```python
from build123d import *

# Parameters (mm, degrees)
SKETCH1_R           = 7.62
BOSS_EXTRUDE1_DEPTH = 2.54
SKETCH2_R           = 6.35
BOSS_EXTRUDE2_DEPTH = 2.54
SKETCH4_R           = 3.175
CUT_EXTRUDE1_DEPTH  = 8.62


with BuildPart() as part:
    # Sketch1 → Boss-Extrude1 (new body)
    with BuildSketch(Plane.XY):
        Circle(SKETCH1_R)
    boss_extrude1 = extrude(amount=BOSS_EXTRUDE1_DEPTH)

    # Sketch2 → Boss-Extrude2 (add)
    with BuildSketch(Plane.XY.offset(2.54)):
        Circle(SKETCH2_R)
    extrude(amount=BOSS_EXTRUDE2_DEPTH)

    # Mirror1: Boss-Extrude1 across plane
    add(boss_extrude1.mirror(Plane.XY.offset(3.81)))

    # Sketch4 → Cut-Extrude1 (cut, through all)
    with BuildSketch(Plane.XY.offset(7.62)):
        Circle(SKETCH4_R)
    extrude(amount=-CUT_EXTRUDE1_DEPTH, mode=Mode.SUBTRACT)


solid = part.part
```
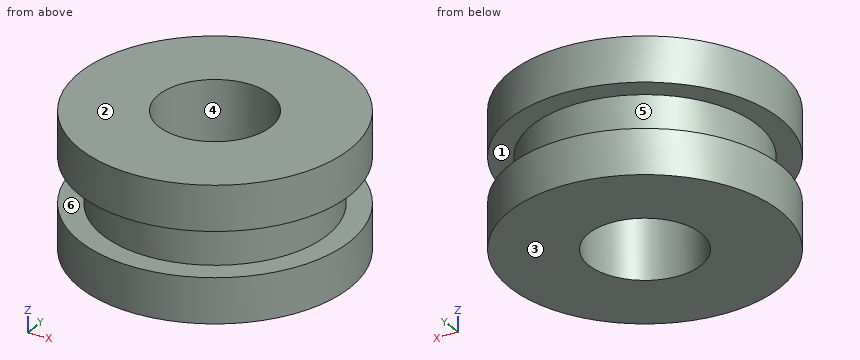
Design review of the part built by this model. Coordinates are the model's own, in mm. Face numbers are marked on the shaded views. A direction names the side the tool comes from. Coordinates: 2 decimals unless noted, no trailing zeros. Write each loop counter-clockwise with the first axis right and the second up, starting at its lowest first coordinate (ties: lowest second). Pieces come first, ordered by that corner, then holes.
1) To check wall thickness, follow L1, parallel to Y at x = 0, z = 4.5 (3 decimals); L2, parallel to X at y = -2.75, z = 2; L3, parallel to Z at x = -1, y = -6.5. State the ranges of each line that lie inside material, in increasing order.
2) Insertion check: pin 1 (3 mm diameter, centred on x = -3.5, z = 4.5, fed in from -Y); pin 2 (3 mm diameter, centred on y = -5, z = 2, fed in from -X); pin 3 (3 mm diameter, centred on y = 5, z = 3, fed in from +X); pin 4 (5 mm diameter, centred on x = 0, y = 0, fed in from +Z). Each pin has a flat end and moves straight along its axis. Give the tip position at first contact, or say it passes through.
3) Add section D-D (y = -5). Write out the cut boundary in (x, z).
4) Mouldability with a two-part tool opening along Z and no side actions: class the marked faces 3, 4, 5 and 6 as +Z half, -Z half, draft (parallel to the pull), parting line (faces both ways), or undercut.
5) Add section C-C (z = 4). Write out the cut boundary in (x, y) (3 decimals).
6) Machinability: for the marked faces 1 and 2, which of the approach directions +Z, -Z, +X, -X, +Y, -Y give a long, thin tool a straight path to every point of the face, cutting with its end or side? Answer none if there is none.
7) Add section A-A (y = 0). Write out the cut boundary in (x, z) (3 decimals).
Check result:
1. L1: y = -6.35 to -3.175, 3.175 to 6.35
1. L2: x = -7.11 to -1.59, 1.59 to 7.11
1. L3: z = 0 to 2.54, 5.08 to 7.62
2. pin 1: stops at y = -7.32
2. pin 2: stops at x = -6.77
2. pin 3: stops at x = 6.73
2. pin 4: passes through
3. outline: (-5.75, 0) - (5.75, 0) - (5.75, 2.54) - (3.91, 2.54) - (3.91, 5.08) - (5.75, 5.08) - (5.75, 7.62) - (-5.75, 7.62) - (-5.75, 5.08) - (-3.91, 5.08) - (-3.91, 2.54) - (-5.75, 2.54) - close
4. face 3: -Z half
4. face 4: draft
4. face 5: undercut
4. face 6: undercut
5. outline: circle Ø12.7 at (0, 0); hole circle Ø6.35 at (0, 0)
6. face 1: none
6. face 2: +Z, +X, -X, +Y, -Y
7. outline: (-7.62, 0) - (-3.175, 0) - (-3.175, 7.62) - (-7.62, 7.62) - (-7.62, 5.08) - (-6.35, 5.08) - (-6.35, 2.54) - (-7.62, 2.54) - close; (3.175, 0) - (7.62, 0) - (7.62, 2.54) - (6.35, 2.54) - (6.35, 5.08) - (7.62, 5.08) - (7.62, 7.62) - (3.175, 7.62) - close
